Design review of the part built by this model. Coordinates are the model's own, in mm. Face numbers are marked on the shaded views. A direction names the side the tool comes from. Give positions to 0.01 mm unless a question says otherwise; leave off trailing zeros. Order: outer loops, then holes, each group sorted by start corner. A loop starts at its lowest first (then second) coordinate and runs counter-clockwise, first axis right, second up. Notation, with made-up numbers: (-20.5, 38.25) -> (17.5, 38.25) arc R25 ccw to (17.5, 53.25) -> close; hole circle Ø5 at (53, 15.5). An arc over 180 degrees is marked (long way). One line per item, written item: value. Start each with the question number.
1) Consider section D-D (x = 0). State the section outline as (y, z) points.
2) Tool access review of the marked faces 1 and 2: name each direction out of +Z, -Z, +X, -X, +Y, -Y from which nothing blocks a thin tool from reaching the whole face with its end or side.
3) Wall thickness on line 1 along Z through (x, y) = (-10.5, 15.5); line 2 along X through (y, z) = (8, 21); line 3 along X through (y, z) = (17.25, -23): over which ranges is each line inside the solid? List them lowest first. Write a range as from..to.
4) The part is to be moulded in two halves that separate along Z. For the marked faces 3, 4, 5 and 6, say which applies: released by +Z, released by -Z, zero draft, split by the parting line, or undercut.
5) Consider section C-C (z = 7.25). State the section outline as (x, y) points.
6) For pin 1 (3 mm diameter, centred on y = 10.5, z = -4.5, fed in from -X); pin 2 (1 mm diameter, centred on x = 7, z = -16.5, fed in from -Y); pin 3 (6 mm diameter, centred on y = 18, z = 23, fed in from +X), all flat-tipped, find the tip position at first contact; note any pin that passes through.
7) Consider section B-B (x = -12.5). State the section outline as (y, z) points, plus the area to 3 significant figures.
8) Consider section A-A (z = -17). State the section outline as (x, y) points, plus the area to 3 significant figures.
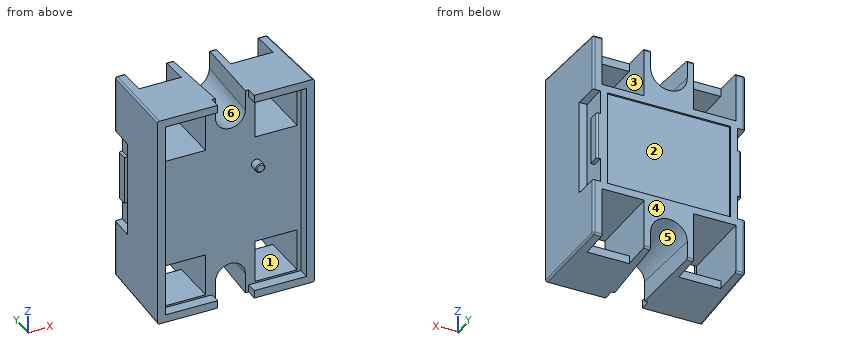
from build123d import *

# Parameters (mm, degrees)
SKETCH1_W           = 41.5
SKETCH1_H           = 57
BOSS_EXTRUDE1_DEPTH = 24
CUT_EXTRUDE1_DEPTH  = 21
CUT_EXTRUDE1_TAPER  = 2.5
SKETCH3_W           = 11.5
SKETCH3_H           = 13.5
CUT_EXTRUDE2_DEPTH  = 8
SKETCH4_W           = 11.5
SKETCH4_H           = 11.5
CUT_EXTRUDE3_DEPTH  = 17.0000001
SKETCH5_W           = 26
SKETCH5_H           = 7
CUT_EXTRUDE4_DEPTH  = 2
SKETCH6_W           = 13
SKETCH6_H           = 3
BOSS_EXTRUDE2_DEPTH = 1
SKETCH7_W           = 33.5
SKETCH7_H           = 26
CUT_EXTRUDE5_DEPTH  = 0.5
SKETCH8_W           = 38.5
SKETCH8_H           = 54
CUT_EXTRUDE6_DEPTH  = 3
SKETCH9_W           = 10
SKETCH9_H           = 3
CUT_EXTRUDE7_DEPTH  = 58.0000001
DRAFT1_ANGLE        = 1.5
FILLET1_R           = 0.5
SKETCH10_R          = 1.25
BOSS_EXTRUDE3_DEPTH = 2.5
CHAMFER1_SIZE       = 0.25


with BuildPart() as part:
    # Sketch1 → Boss-Extrude1 (new body)
    with BuildSketch(Plane(origin=(0, 0, 0), x_dir=(1, 0, 0), z_dir=(0, 1, 0))):
        Rectangle(SKETCH1_W, SKETCH1_H)
    extrude(amount=BOSS_EXTRUDE1_DEPTH)

    # Sketch2 → Cut-Extrude1 (cut)
    with BuildSketch(Plane(origin=(0, 24, 0), x_dir=(1, 0, 0), z_dir=(0, 1, 0))):
        with BuildLine():
            Line((-5, -23.5), (-5, -30.5))
            Line((-5, -30.5), (5, -30.5))
            Line((5, -30.5), (5, -23.5))
            ThreePointArc((5, -23.5), (0, -18.5), (-5, -23.5))
        make_face()
    cut_extrude1 = extrude(amount=-CUT_EXTRUDE1_DEPTH, taper=CUT_EXTRUDE1_TAPER, mode=Mode.SUBTRACT)

    # Sketch3 → Cut-Extrude2 (cut)
    with BuildSketch(Plane(origin=(0, 24, 0), x_dir=(1, 0, 0), z_dir=(0, 1, 0))):
        with Locations((-12.5, -21.75)):
            Rectangle(SKETCH3_W, SKETCH3_H)
        with Locations((12.5, -21.75)):
            Rectangle(SKETCH3_W, SKETCH3_H)
    cut_extrude2 = extrude(amount=-CUT_EXTRUDE2_DEPTH, mode=Mode.SUBTRACT)

    # Sketch4 → Cut-Extrude3 (cut, through all)
    with BuildSketch(Plane(origin=(0, 16, 0), x_dir=(1, 0, 0), z_dir=(0, 1, 0))):
        with Locations((-12.5, -20.75)):
            Rectangle(SKETCH4_W, SKETCH4_H)
        with Locations((12.5, -20.75)):
            Rectangle(SKETCH4_W, SKETCH4_H)
    cut_extrude3 = extrude(amount=-CUT_EXTRUDE3_DEPTH, mode=Mode.SUBTRACT)

    # Mirror1: Cut-Extrude1, Cut-Extrude2, Cut-Extrude3 across plane
    add(cut_extrude1.mirror(Plane.XY), mode=Mode.SUBTRACT)
    add(cut_extrude2.mirror(Plane.XY), mode=Mode.SUBTRACT)
    add(cut_extrude3.mirror(Plane.XY), mode=Mode.SUBTRACT)

    # Sketch5 → Cut-Extrude4 (cut)
    with BuildSketch(Plane.ZY.offset(20.75)):
        with Locations((0, 20.5)):
            Rectangle(SKETCH5_W, SKETCH5_H)
    cut_extrude4 = extrude(amount=-CUT_EXTRUDE4_DEPTH, mode=Mode.SUBTRACT)

    # Sketch6 → Boss-Extrude2 (add)
    with BuildSketch(Plane.ZY.offset(18.75)):
        with Locations((0, 22.5)):
            Rectangle(SKETCH6_W, SKETCH6_H)
    boss_extrude2 = extrude(amount=BOSS_EXTRUDE2_DEPTH)

    # Mirror2: Cut-Extrude4, Boss-Extrude2 across plane
    add(cut_extrude4.mirror(Plane(origin=(0, 0, 0), x_dir=(0, 0, 1), z_dir=(1, 0, 0))), mode=Mode.SUBTRACT)
    add(boss_extrude2.mirror(Plane(origin=(0, 0, 0), x_dir=(0, 0, 1), z_dir=(1, 0, 0))))

    # Sketch7 → Cut-Extrude5 (cut)
    with BuildSketch(Plane(origin=(0, 24, 0), x_dir=(1, 0, 0), z_dir=(0, 1, 0))):
        Rectangle(SKETCH7_W, SKETCH7_H)
    extrude(amount=-CUT_EXTRUDE5_DEPTH, mode=Mode.SUBTRACT)

    # Sketch8 → Cut-Extrude6 (cut)
    with BuildSketch(Plane.XZ):
        Rectangle(SKETCH8_W, SKETCH8_H)
    extrude(amount=-CUT_EXTRUDE6_DEPTH, mode=Mode.SUBTRACT)

    # Sketch9 → Cut-Extrude7 (cut, through all)
    with BuildSketch(Plane(origin=(0, 0, -28.5), x_dir=(-1, 0, 0), z_dir=(0, 0, -1))):
        with Locations((0, 1.5)):
            Rectangle(SKETCH9_W, SKETCH9_H)
    extrude(amount=-CUT_EXTRUDE7_DEPTH, mode=Mode.SUBTRACT)

    # Draft1
    draft1_faces = [part.faces().sort_by_distance(p)[0] for p in [
        (-12.725295126, 9.445247328, -28.5),
        (12.725295126, 9.445247328, -28.5),
        (-20.75, 10.695615514, 0),
        (-12.725295126, 9.445247328, 28.5),
        (12.725295126, 9.445247328, 28.5),
        (20.75, 10.695615514, 0),
    ]]
    draft(draft1_faces, Plane.ZX.offset(24), DRAFT1_ANGLE)

    # Fillet1
    fillet1_edges = [part.edges().sort_by_distance(p)[0] for p in [
        (-20.75, 24, -20.75),
        (-19.5, 24, -28.5),
        (5.875, 24, -28.5),
        (-19.5, 24, 28.5),
        (5.875, 24, 28.5),
        (-20.75, 24, 20.75),
        (-19.75, 24, 0),
        (20.75, 24, -20.75),
        (19.75, 24, 0),
        (-5.875, 24, 28.5),
        (20.75, 24, 20.75),
        (19.5, 24, 28.5),
        (19.5, 24, -28.5),
        (21.064231059, 12, 28.814231059),
        (-21.064231059, 12, 28.814231059),
        (-21.064231059, 12, -28.814231059),
        (21.064231059, 12, -28.814231059),
        (-5.875, 24, -28.5),
    ]]
    fillet(fillet1_edges, radius=FILLET1_R)

    # Sketch10 → Boss-Extrude3 (add)
    with BuildSketch(Plane.XZ.offset(-3)):
        with Locations((7, 7.25)):
            Circle(SKETCH10_R)
    extrude(amount=BOSS_EXTRUDE3_DEPTH)

    # Chamfer1
    chamfer1_edges = [part.edges().sort_by_distance(p)[0] for p in [
        (5.75, 0.5, 7.25),
    ]]
    chamfer(chamfer1_edges, length=CHAMFER1_SIZE)


solid = part.part
Checked values:
1. outline: (3, -19.42) -> (24, -18.5) -> (24, -13) -> (23.5, -13) -> (23.5, 13) -> (24, 13) -> (24, 18.5) -> (3, 19.42) -> close
2. face 1: +Y, -Y
2. face 2: +Y
3. line 1: z = -28.72..-26.5, -15..15, 26.5..28.72
3. line 2: x = -21.17..-18.25, -6.75..-3.5, 3.5..6.75, 18.25..21.17
3. line 3: x = -20.93..-18.25, -6.75..-4.68, 4.68..6.75, 18.25..20.93
4. face 3: undercut
4. face 4: zero draft
4. face 5: released by -Z
4. face 6: released by +Z
5. outline: (-21.38, 0) -> (-19.25, 0) -> (-19.25, 3) -> (5.75, 3) -> (5.75, 0.75) -> (6, 0.5) -> (8, 0.5) -> (8.25, 0.75) -> (8.25, 3) -> (19.25, 3) -> (19.25, 0) -> (21.38, 0) -> (20.93, 17) -> (18.75, 17) -> (18.75, 24) -> (16.75, 24) -> (16.75, 23.5) -> (-16.75, 23.5) -> (-16.75, 24) -> (-18.75, 24) -> (-18.75, 17) -> (-20.93, 17) -> close
6. pin 1: stops at x = -21.14
6. pin 2: stops at y = 3
6. pin 3: stops at x = 20.99
7. outline: (0, -29.13) -> (16, -28.71) -> (16, -26.5) -> (3, -26.5) -> (3, -27) -> (0, -27) -> close; (0, 27) -> (3, 27) -> (3, 26.5) -> (16, 26.5) -> (16, 28.71) -> (0, 29.13) -> close; (3, -15) -> (24, -15) -> (24, -13) -> (23.5, -13) -> (23.5, 13) -> (24, 13) -> (24, 15) -> (3, 15) -> close
7. area: 691 mm^2
8. outline: (-21.38, 0) -> (-19.25, 0) -> (-19.25, 3) -> (-18.25, 3) -> (-18.25, 24) -> (-20.26, 24) arc R0.5 ccw to (-20.76, 23.51) -> close; (-6.75, 3) -> (6.75, 3) -> (6.75, 24) -> (-6.75, 24) -> close; (18.25, 3) -> (19.25, 3) -> (19.25, 0) -> (21.38, 0) -> (20.76, 23.51) arc R0.5 ccw to (20.26, 24) -> (18.25, 24) -> close
8. area: 412 mm^2
